Read the model definition and answer for the solid it produces. Units are mm, in the model's axes. Round coordinates to 2 decimals unless told otherwise and drop trailing zeros. Write each loop counter-clockwise with the first axis right and the second up, starting at its lowest first coordinate (ties: lowest second). Pieces come first, ordered by that corner, then holes. Notation, with made-up numbers: (14, 60.5) - (35, 60.5) arc R21 cw to (35, 96.5) - close; hole circle Ø11 at (-9, 71.25). An arc over 180 degrees is marked (long way). Use one line per item in the form item = value. Start each with the question number.
1) The part is cut by section A-A, the plane x = -2. Give the vertices of the cut face in (y, z).
2) The part is cut by section B-B, the plane y = 2.75. Give the vertices of the cut face in (x, z), plus the area to 3 significant figures.
3) Consider line 1 along Y through (x, z) = (-9, 0); line 2 along Y through (x, z) = (-6.5, 0); line 3 along Y through (x, z) = (-8, 0). Determine where each line is inside the solid, lowest interval first. Write a range as from..to.
4) The part is cut by section C-C, the plane x = -8.75. Give the vertices of the cut face in (y, z), plus the area to 3 significant figures.
5) The part is cut by section D-D, the plane y = 13.75. Give the vertices of the cut face in (x, z), plus the area to 3 significant figures.
6) This flat-tipped pin is pushed along its axis until it touches: pin 1 (3 mm diameter, centred on x = -5, y = 3, fed in from -Z). Where does it stop, or does it pass through?
from build123d import *

# Parameters (mm, degrees)
BOSS_EXTRUDE1_DEPTH     = 0.12
CUT_EXTRUDE1_DEPTH      = 22.096388316
CUT_EXTRUDE1_DEPTH_BACK = 22.096388316
SKETCH3_RX              = 3
SKETCH3_RY              = 0.5
SKETCH3_W               = 2
SKETCH3_H               = 2
FILLET1_R               = 0.7


with BuildPart() as part:
    # Sketch1 → Boss-Extrude1 (new, symmetric)
    with BuildSketch(Plane.XY):
        Polygon((0, 0), (-11, 0), (-11, 11), (-11, 18), (0, 18), (0, 11), align=None)
        Polygon((-1, 1), (-1, 6), (-3, 6), (-3, 5.5), (-4.5, 5.5), (-4.5, 6.5), (-5.5, 6.5), (-5.5, 8), (-5, 8), (-5, 10), (-10, 10), (-10, 1), align=None, mode=Mode.SUBTRACT)
    extrude(amount=BOSS_EXTRUDE1_DEPTH, both=True)

    # Sketch3 → Cut-Extrude1 (cut, two sides: drawn at the far end of the back side and taken through both)
    with BuildSketch(Plane.XY.offset(0.12).offset(-CUT_EXTRUDE1_DEPTH_BACK)):
        with Locations(Location((-5.5, 16.75), (0, 0, 180))):
            Ellipse(SKETCH3_RX, SKETCH3_RY)
        Polygon((-10, 11), (-5, 11), (-6.5, 15.25), (-10, 15.25), align=None)
        Polygon((-1, 11), (-1, 15.25), (-4.5, 15.25), (-3, 11), align=None)
        with Locations((-2, 9)):
            Rectangle(SKETCH3_W, SKETCH3_H)
    extrude(amount=CUT_EXTRUDE1_DEPTH + CUT_EXTRUDE1_DEPTH_BACK, mode=Mode.SUBTRACT)

    # Fillet1
    fillet1_edges = [part.edges().sort_by_distance(p)[0] for p in [
        (-1, 6, 0),
        (-5, 10, 0),
        (-1, 10, 0),
        (-1, 8, 0),
        (-3, 8, 0),
        (-3, 10, 0),
        (-4.5, 15.25, 0),
        (-1, 15.25, 0),
        (-1, 11, 0),
        (-3, 11, 0),
        (-10, 11, 0),
        (-10, 15.25, 0),
        (-6.5, 15.25, 0),
        (-5, 11, 0),
    ]]
    fillet(fillet1_edges, radius=FILLET1_R)


solid = part.part
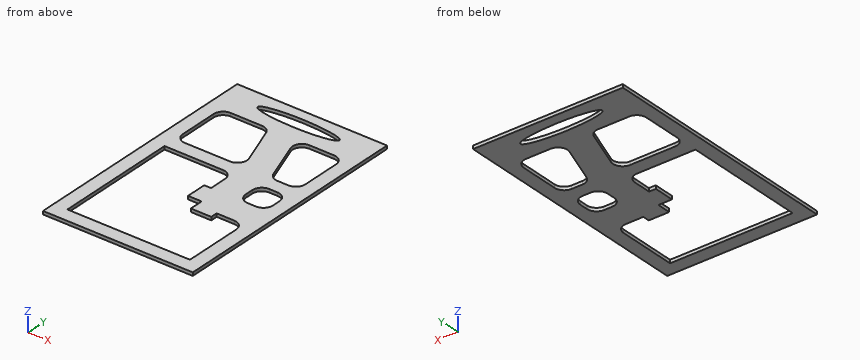
Geometry results:
q1.outline = (0, -0.12) - (1, -0.12) - (1, 0.12) - (0, 0.12) - close; (6, -0.12) - (8, -0.12) - (8, 0.12) - (6, 0.12) - close; (10, -0.12) - (11, -0.12) - (11, 0.12) - (10, 0.12) - close; (15.25, -0.12) - (18, -0.12) - (18, 0.12) - (15.25, 0.12) - close
q2.outline = (-11, -0.12) - (-10, -0.12) - (-10, 0.12) - (-11, 0.12) - close; (-1, -0.12) - (0, -0.12) - (0, 0.12) - (-1, 0.12) - close
q2.area = 0.480 mm2
q3.line_1 = 0..1, 10..11, 15.25..18
q3.line_2 = 0..1, 10..11, 15.04..16.28, 17.22..18
q3.line_3 = 0..1, 10..11, 15.25..16.47, 17.03..18
q4.outline = (0, -0.12) - (1, -0.12) - (1, 0.12) - (0, 0.12) - close; (10, -0.12) - (11, -0.12) - (11, 0.12) - (10, 0.12) - close; (15.25, -0.12) - (18, -0.12) - (18, 0.12) - (15.25, 0.12) - close
q4.area = 1.14 mm2
q5.outline = (-11, -0.12) - (-10, -0.12) - (-10, 0.12) - (-11, 0.12) - close; (-5.97, -0.12) - (-3.97, -0.12) - (-3.97, 0.12) - (-5.97, 0.12) - close; (-1, -0.12) - (0, -0.12) - (0, 0.12) - (-1, 0.12) - close
q5.area = 0.960 mm2
q6.pin_1 = through
